from build123d import *

# Parameters (mm, degrees)
F0_R     = 7.2
F0_R_2   = 1.25
F1_DEPTH = 3.5
F2_R     = 7.2
F2_R_2   = 5.75
F3_DEPTH = 15
F4_R     = 1


with BuildPart() as f1:
    # F0 (on Top) → F1 (new body)
    with BuildSketch(Plane.XY):
        Circle(F0_R)
        Circle(F0_R_2, mode=Mode.SUBTRACT)
    extrude(amount=F1_DEPTH)

    # F2 (on Top) → F3 (join)
    with BuildSketch(Plane.XY):
        Circle(F2_R)
        Circle(F2_R_2, mode=Mode.SUBTRACT)
    extrude(amount=F3_DEPTH)

    # F4
    f4_edges = [f1.edges().sort_by_distance(p)[0] for p in [
        (-7.2, 0, 0),
        (-5.75, 0, 15),
    ]]
    fillet(f4_edges, radius=F4_R)


solid = f1.part
Work out the finished part from the listing and answer in its coordinate system (mm). A direction names the side the tool comes from. Give positions to 0.01 mm unless a question says otherwise; leave off trailing zeros. Loops run counter-clockwise (first coordinate to the right, second up) from the corner with the lowest first, then second, coordinate; pieces in that order, holes last. Notation, with made-up numbers: (-2, -33) - (4, -33) arc R5 ccw to (4, -28) - close; hole circle Ø11 at (34, 27). An arc over 180 degrees is marked (long way). Answer in a Markdown table with one row per item.
(1) Section A-A (y = 0) is taken. Give the vertices of the cut face in (x, z), and give its area (3 significant figures).
Results list:
| item | result |
|---|---|
| outline | (-7.2, 1) arc R1 ccw to (-6.2, 0) - (-1.25, 0) - (-1.25, 3.5) - (-5.75, 3.5) - (-5.75, 14) arc R1 ccw to (-6.75, 15) - (-7.2, 15) - close; (1.25, 0) - (6.2, 0) arc R1 ccw to (7.2, 1) - (7.2, 15) - (6.75, 15) arc R1 ccw to (5.75, 14) - (5.75, 3.5) - (1.25, 3.5) - close |
| area | 74.1 mm² |
(2) Consider L1, parallel to Y at x = 0, z = 8.5; L2, parallel to Z at x = 1.5, y = -5; L3, parallel to Y at x = 2.75, z = 14.25. Determine where each line is inside the solid, lowest interval first. Write a range as [from, to].
Results list:
| item | result |
|---|---|
| L1 | y = [-7.2, -5.75], [5.75, 7.2] |
| L2 | z = [0, 3.5] |
| L3 | y = [-6.65, -5.09], [5.09, 6.65] |
(3) For a pull along Y with two mould halves and no side action, classify faces 3 (the face through (6.87, 2.16, 7.9)), 4 (the face through (-0.1, 1.4, 3.5)), 5 (the face through (-0.1, 1.5, 0)) as pulls with the +Y half, pulls with the -Y half, needs draft (parallel to the pull), parting line crosses it, or undercut.
Results list:
| item | result |
|---|---|
| face 3 | parting line crosses it |
| face 4 | undercut |
| face 5 | needs draft |
(4) Section D-D (z = 1.5) is taken. Give the vertices of the cut face in (x, y).
Results list:
| item | result |
|---|---|
| outline | circle Ø14.4 at (0, 0); hole circle Ø2.5 at (0, 0) |
(5) Flat-ended cylindrical pins translate along their axes: pin 1 Ø8 at (x, z) = (-5.5, 3) entering from +Y; pin 2 Ø4 at (y, z) = (5.5, 4) entering from -X; pin 3 Ø1.5 at (x, y) = (3.5, 3) entering from +Z; pin 4 Ø1.5 at (x, y) = (0, 0) entering from +Z. Find the tip coordinate at first contact, or state that the pin passes through.
Results list:
| item | result |
|---|---|
| pin 1 | stops at y = 7.04 |
| pin 2 | stops at x = -6.29 |
| pin 3 | stops at z = 3.5 |
| pin 4 | passes through |
(6) Section C-C (z = 13) is taken. Give the vertices of the cut face in (x, y).
Results list:
| item | result |
|---|---|
| outline | circle Ø14.4 at (0, 0); hole circle Ø11.5 at (0, 0) |
(7) A tool of negligible diameter and unlimited length cuts with its end or side. For faces 1 (the face through (-0.75, 5.7, 8.68)), 2 (the face through (-0.27, -1.22, 1.73)), from which of +Z, -Z, +X, -X, +Y, -Y can it reach the whole face along a straight path? Write none if from no direction.
Results list:
| item | result |
|---|---|
| face 1 | +Z |
| face 2 | +Z, -Z |
